Input: part model. Units: mm. Frame: model coordinates. Coordinates: 2 decimals unless noted, no trailing zeros. Order: outer loops, then holes, each group sorted by start corner. A loop starts at its lowest first (then second) coordinate and runs counter-clockwise, first axis right, second up. Notation, with made-up numbers: M 2.5,6.25 L 54.5,6.25 A34 ccw 54.5,36.25 Z; hole C 65.25,7 d2. An arc over 180 degrees is marked long. Answer in a Markdown table with one row per item.
from build123d import *

# Parameters (mm, degrees)
SKETCH1_R                                       = 2.6
SKETCH1_R_2                                     = 2.7
BOSS_EXTRUDE1_DEPTH                             = 6
FILLET1_R                                       = 7.5
CSK_FOR_M5_FLAT_HEAD_MACHINE_SCREW1_D           = 5.5
CSK_FOR_M5_FLAT_HEAD_MACHINE_SCREW1_CSINK_D     = 10.4
CSK_FOR_M5_FLAT_HEAD_MACHINE_SCREW1_CSINK_ANGLE = 90


with BuildPart() as part:
    # Sketch1 → Boss-Extrude1 (new body)
    with BuildSketch(Plane(origin=(0, 0, 0), x_dir=(1, 0, 0), z_dir=(0, 1, 0))):
        with BuildLine():
            Line((31.883633055, 20.164562188), (44.561021943, 28.182280752))
            ThreePointArc((44.561021943, 28.182280752), (52.725, 0), (44.561021943, -28.182280752))
            Line((44.561021943, -28.182280752), (31.883633055, -20.164562188))
            ThreePointArc((31.883633055, -20.164562188), (0, -37.725), (-31.883633055, -20.164562188))
            Line((-31.883633055, -20.164562188), (-44.561021943, -28.182280752))
            ThreePointArc((-44.561021943, -28.182280752), (-52.725, 0), (-44.561021943, 28.182280752))
            Line((-44.561021943, 28.182280752), (-31.883633055, 20.164562188))
            ThreePointArc((-31.883633055, 20.164562188), (0, 37.725), (31.883633055, 20.164562188))
        make_face()
        with Locations(Location((-11.083898795, 11.083898795, 0), (0, 0, 270))):
            Circle(SKETCH1_R, mode=Mode.SUBTRACT)
        with Locations(Location((11.083898795, 11.083898795, 0), (0, 0, 270))):
            Circle(SKETCH1_R, mode=Mode.SUBTRACT)
        with Locations(Location((11.083898795, -11.083898795, 0), (0, 0, 270))):
            Circle(SKETCH1_R, mode=Mode.SUBTRACT)
        with Locations(Location((-11.083898795, -11.083898795, 0), (0, 0, 270))):
            Circle(SKETCH1_R, mode=Mode.SUBTRACT)
        with Locations(Location((41.701925915, 17.5, 0), (0, 0, 270))):
            Circle(SKETCH1_R_2, mode=Mode.SUBTRACT)
        with Locations(Location((41.701925915, -17.5, 0), (0, 0, 270))):
            Circle(SKETCH1_R_2, mode=Mode.SUBTRACT)
        with Locations(Location((-41.701925915, 17.5, 0), (0, 0, 90))):
            Circle(SKETCH1_R_2, mode=Mode.SUBTRACT)
        with Locations(Location((-41.701925915, -17.5, 0), (0, 0, 90))):
            Circle(SKETCH1_R_2, mode=Mode.SUBTRACT)
    extrude(amount=BOSS_EXTRUDE1_DEPTH)

    # Fillet1
    fillet1_edges = [part.edges().sort_by_distance(p)[0] for p in [
        (44.561021943, 3, 28.182280752),
        (31.883633055, 3, 20.164562188),
        (-44.561021943, 3, 28.182280752),
        (-31.883633055, 3, 20.164562188),
        (44.561021943, 3, -28.182280752),
        (31.883633055, 3, -20.164562188),
        (-44.561021943, 3, -28.182280752),
        (-31.883633055, 3, -20.164562188),
    ]]
    fillet(fillet1_edges, radius=FILLET1_R - 0.0001)  # a hair under: the kernel refuses the full size

    # CSK for M5 Flat Head Machine Screw1 (through all)
    with Locations(Plane(origin=(0, 6, 0), x_dir=(1, 0, 0), z_dir=(0, 1, 0))):
        with Locations((-11.083898795, 11.083898795), (11.083898795, 11.083898795), (11.083898795, -11.083898795), (-11.083898795, -11.083898795)):
            CounterSinkHole(CSK_FOR_M5_FLAT_HEAD_MACHINE_SCREW1_D / 2, CSK_FOR_M5_FLAT_HEAD_MACHINE_SCREW1_CSINK_D / 2, counter_sink_angle=CSK_FOR_M5_FLAT_HEAD_MACHINE_SCREW1_CSINK_ANGLE)


solid = part.part
1) Cut plane D-D, the plane x = 32. Output: boundary loops of the cut face in (y, z), and give its area (3 significant figures).
Resolved:
| item | result |
|---|---|
| outline | M 0,-22.87 L 6,-22.87 L 6,22.87 L 0,22.87 Z |
| area | 274 mm2 |
2) Contact query for flat-ended pins moving along their axis: pin 1 (5 mm diameter, centred on x = 11.08, z = -11.08, fed in from -Y); pin 2 (1 mm diameter, centred on y = 2.5, z = -9, fed in from -X); pin 3 (1.5 mm diameter, centred on y = 3.5, z = -17.5, fed in from +X); pin 4 (7 mm diameter, centred on x = -11.08, z = 11.08, fed in from +Y). Output: stop coordinate, or through.
Resolved:
| item | result |
|---|---|
| pin 1 | passes through |
| pin 2 | stops at x = -52.04 |
| pin 3 | stops at x = 49.99 |
| pin 4 | stops at y = 4.31 |
3) Cut plane B-B, the plane y = 2.25. State how many separate pieces and enclosed holes the cut face has, and give its area (3 significant figures).
Resolved:
| item | result |
|---|---|
| separate pieces | 1 |
| enclosed holes | 8 |
| area | 5,790 mm2 |
4) Cut plane A-A, the plane z = 17.5. Output: boundary loops of the cut face in (x, y).
Resolved:
| item | result |
|---|---|
| outline | M -49.74,0 L -44.4,0 L -44.4,6 L -49.74,6 Z; M -39,0 L 39,0 L 39,6 L -39,6 Z; M 44.4,0 L 49.74,0 L 49.74,6 L 44.4,6 Z |
5) Material intervals for probe 1 along X at (y, z) = (3.9, 17.5); probe 2 along X at (y, z) = (2.35, -11); probe 3 along Z at (x, y) = (13, 3.75), sorted ascending.
Resolved:
| item | result |
|---|---|
| probe 1 | x = -49.74 to -44.4, -39 to 39, 44.4 to 49.74 |
| probe 2 | x = -51.56 to -13.83, -8.34 to 8.34, 13.83 to 51.56 |
| probe 3 | z = -35.41 to -13.33, -8.84 to 8.84, 13.33 to 35.41 |
6) Mould query, pull axis X, two halves, no side actions, for faces 1 (the face through (1, 6, -1)), 2 (the face through (-52.724, 2.958, 0.293)), 3 (the face through (32.72, 3.04, -22.74)). Classes: +X half, -X half, draft (parallel to the pull), parting line (faces both ways), or undercut.
Resolved:
| item | result |
|---|---|
| face 1 | draft |
| face 2 | -X half |
| face 3 | undercut |
